```python
from build123d import *

# Parameters (mm, degrees)
CROQUIS2_W              = 20
CROQUIS2_H              = 28
SALIENTE_EXTRUIR1_DEPTH = 8
CROQUIS3_W              = 6.705751287
CROQUIS3_H              = 20
CORTAR_EXTRUIR1_DEPTH   = 6
CORTAR_EXTRUIR2_DEPTH   = 5
CROQUIS6_R              = 1.6
CORTAR_EXTRUIR3_DEPTH   = 3
REDONDEO1_R             = 1
SKETCH1_R               = 1.75
CUT_EXTRUDE1_DEPTH      = 24.126770256


with BuildPart() as part:
    # Croquis2 → Saliente-Extruir1 (new body)
    with BuildSketch(Plane(origin=(0, 0, 0), x_dir=(1, 0, 0), z_dir=(0, 1, 0))):
        with Locations((-0.843373494, -5.526104418)):
            Rectangle(CROQUIS2_W, CROQUIS2_H)
    extrude(amount=SALIENTE_EXTRUIR1_DEPTH)

    # Croquis3 → Cortar-Extruir1 (cut)
    with BuildSketch(Plane(origin=(0, 8, 0), x_dir=(1, 0, 0), z_dir=(0, 1, 0))):
        with Locations((5.803750863, -5.526104418)):
            Rectangle(CROQUIS3_W, CROQUIS3_H)
    extrude(amount=-CORTAR_EXTRUIR1_DEPTH, mode=Mode.SUBTRACT)

    # Croquis5 → Cortar-Extruir2 (cut)
    with BuildSketch(Plane(origin=(0, 8, 0), x_dir=(1, 0, 0), z_dir=(0, 1, 0))):
        with BuildLine():
            Line((2.450875219, -15.026104418), (2.450875219, 3.973895582))
            ThreePointArc((2.450875219, 3.973895582), (2.020425803, 3.959111389), (1.589976387, 3.973895582))
            ThreePointArc((1.589976387, 3.973895582), (-1.912953919, 5.345273007), (-4.00171373, 8.473895582))
            Line((-4.00171373, 8.473895582), (-10.843373494, 8.473895582))
            Line((-10.843373494, 8.473895582), (-10.843373494, -19.526104418))
            Line((-10.843373494, -19.526104418), (-4.00171373, -19.526104418))
            ThreePointArc((-4.00171373, -19.526104418), (-1.912953919, -16.397481842), (1.589976387, -15.026104418))
            ThreePointArc((1.589976387, -15.026104418), (2.020425803, -15.011320225), (2.450875219, -15.026104418))
        make_face()
    extrude(amount=-CORTAR_EXTRUIR2_DEPTH, mode=Mode.SUBTRACT)

    # Croquis6 → Cortar-Extruir3 (cut)
    with BuildSketch(Plane(origin=(0, 3, 0), x_dir=(1, 0, 0), z_dir=(0, 1, 0))):
        with Locations(Location((-7.343373494, -5.526104418, 0), (0, 0, 270))):
            Circle(CROQUIS6_R)
    extrude(amount=-CORTAR_EXTRUIR3_DEPTH, mode=Mode.SUBTRACT)

    # Redondeo1
    redondeo1_edges = [part.edges().sort_by_distance(p)[0] for p in [
        (-10.843373494, 1.5, -8.473895582),
        (-10.843373494, 1.5, 19.526104418),
        (-4.00171373, 5.5, 19.526104418),
        (-4.00171373, 5.5, -8.473895582),
        (9.156626506, 4, -8.473895582),
        (9.156626506, 4, 19.526104418),
    ]]
    fillet(redondeo1_edges, radius=REDONDEO1_R)

    # Sketch1 → Cut-Extrude1 (cut, through all)
    with BuildSketch(Plane(origin=(0, 2, 0), x_dir=(1, 0, 0), z_dir=(0, 1, 0))):
        with Locations(Location((5.450875219, -1.026104418, 0), (0, 0, 270))):
            Circle(SKETCH1_R)
        with Locations(Location((5.450875219, -10.026104418, 0), (0, 0, 270))):
            Circle(SKETCH1_R)
    extrude(amount=-CUT_EXTRUDE1_DEPTH, mode=Mode.SUBTRACT)


solid = part.part
```
CAD build for the part. Positions are in the model's coordinates, mm. A direction names the side the tool comes from. Coordinates: 2 decimals unless noted, no trailing zeros. Order: outer loops, then holes, each group sorted by start corner. A loop starts at its lowest first (then second) coordinate and runs counter-clockwise, first axis right, second up.
(1) Saw through at A-A, the plane z = 4.5. Write the cut outline in (x, y), and give its area (3 significant figures).
Solution:
outline: (-10.84, 0) - (-8.57, 0) - (-8.57, 3) - (-10.84, 3) - close; (-6.12, 0) - (9.16, 0) - (9.16, 2) - (2.45, 2) - (2.45, 3) - (-6.12, 3) - close
area: 45.9 mm2
(2) Drill centre lines: L1, parallel to Z at x = 3.5, y = 2.25; L2, parallel to Z at x = 1.5, y = 3.75; L3, parallel to Y at x = -9, z = -3.5. Where is each one in solid material? Low to high.
Solution:
L1: z = -8.47 to -4.47, 15.53 to 19.53
L2: z = -8.47 to -3.98, 15.03 to 19.53
L3: y = 0 to 3
(3) Mould opens along Z. For faces 1 (the face through (9.157, 1, 6)), 2 (the face through (5.528, 1.014, 8.278)), 3 (the face through (1, 3, -8.474)) say: released by +Z, released by -Z, zero draft, split by the parting line, or undercut.
Solution:
face 1: zero draft
face 2: undercut
face 3: released by -Z
(4) Pin check, flat tips, straight feed: pin 1 Ø7.5 at (x, z) = (7.5, 4.5) entering from +Y; pin 2 Ø6 at (x, z) = (4, 6) entering from +Y. Stop position of each tip, or through.
Solution:
pin 1: stops at y = 2
pin 2: stops at y = 3
(5) Saw through at B-B, the plane x = 6.75. Write the cut outline in (y, z), and give its area (3 significant figures).
Solution:
outline: (0, -8.47) - (8, -8.47) - (8, -4.47) - (2, -4.47) - (2, -0.15) - (0, -0.15) - close; (0, 2.2) - (2, 2.2) - (2, 8.85) - (0, 8.85) - close; (0, 11.2) - (2, 11.2) - (2, 15.53) - (8, 15.53) - (8, 19.53) - (0, 19.53) - close
area: 94.6 mm2
(6) Which spindle directions (+Z, -Z, +X, -X, +Y, -Y) get a long thin tool onto all of the face, cutting with end or side? Do faces 4 (the face through (4.781, 1.014, 2.643)), 5 (the face through (-3.339, 5.465, -7.975)), 6 (the face through (6, 5, 15.526)). Say none if no direction does.
Solution:
face 4: +Y, -Y
face 5: -X, +Y
face 6: +X, +Y
(7) Saw through at D-D, the plane x = 2.75. Write the cut outline in (y, z).
Solution:
outline: (0, -8.47) - (8, -8.47) - (8, -4.47) - (2, -4.47) - (2, 15.53) - (8, 15.53) - (8, 19.53) - (0, 19.53) - close
(8) Saw through at C-C, the plane y = 6. Write the cut outline in (x, z), and give its area (3 significant figures).
Solution:
outline: (-3.33, -6.95) arc R1 ccw to (-2.47, -8.47) - (8.16, -8.47) arc R1 ccw to (9.16, -7.47) - (9.16, -4.47) - (2.45, -4.47) - (2.45, -3.97) arc R6.27 ccw to start; (-3.33, 18) arc R6.27 ccw to (2.45, 15.03) - (2.45, 15.53) - (9.16, 15.53) - (9.16, 18.53) arc R1 ccw to (8.16, 19.53) - (-2.47, 19.53) arc R1 ccw to start
area: 96.0 mm2
